Job drawing, mm, ordinate dimensions from the low corner. One solid piece. Coordinates: 2 decimals unless noted, no trailing zeros. Loops run counter-clockwise (first coordinate to the right, second up) from the corner with the lowest first, then second, coordinate; pieces in that order, holes last. Notation, with made-up numbers: (-27.5, 6.25) -> (-21.5, 6.25) arc R32 cw to (-21.5, 37.25) -> close; hole circle Ø3 at (71.5, -32). An arc over 180 degrees is marked (long way). Use one line per item in the form item = value. Start each with the question number.
(1) Band-saw the part on B-B on y = 12. Give the cut face in (x, z).
(2) Band-saw the part on A-A on z = 0.5. Give the cut face in (x, y).
(3) Band-saw the part on C-C on x = 6.5. Give the cut face in (y, z).
(4) Drill centre lines: L1, parallel to X at y = 14.5, z = 1.75; L2, parallel to Y at x = 30, z = 0.55. Where is each one in solid material? Low to high. Write a range as [from, to].
(5) Pin check, flat tips, straight feed: P1, Ø1.1, axis at x = 36.5, z = 1.5, coming from the +Y side; P2, Ø1.1, axis at y = 12.5, z = 0.5, coming from the +X side. Stop position of each tip, or through.
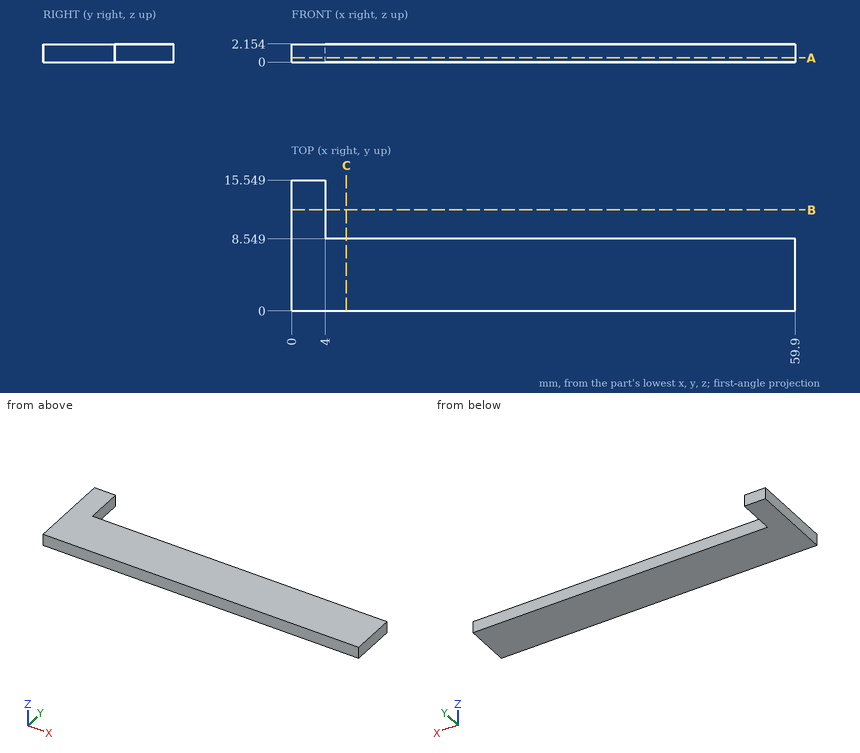
A:
q1.outline = (0, 0) -> (4, 0) -> (4, 2.15) -> (0, 2.15) -> close
q2.outline = (0, 0) -> (59.9, 0) -> (59.9, 8.55) -> (4, 8.55) -> (4, 15.55) -> (0, 15.55) -> close
q3.outline = (0, 0) -> (8.55, 0) -> (8.55, 2.15) -> (0, 2.15) -> close
q4.L1 = [0, 4]
q4.L2 = [0, 8.55]
q5.P1 = 8.55
q5.P2 = 4
